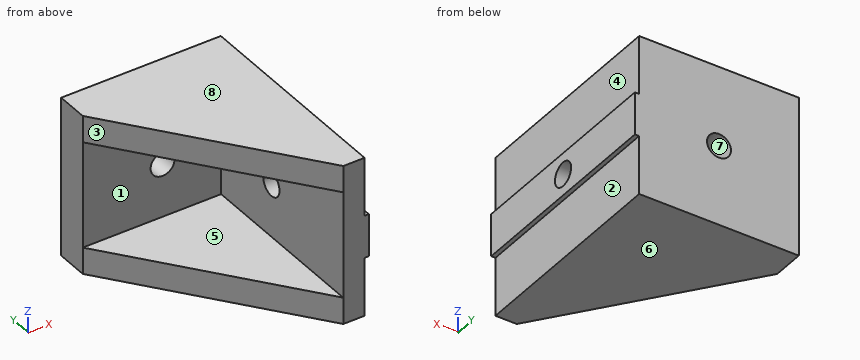
from build123d import *

# Parameters (mm, degrees)
BOSS_EXTRUDE1_DEPTH = 15
SKETCH2_W           = 8
SKETCH2_H           = 40
BOSS_EXTRUDE2_DEPTH = 0.8
SKETCH3_W           = 26
SKETCH3_H           = 34
CUT_EXTRUDE1_DEPTH  = 10
SKETCH4_R           = 2.25
CUT_EXTRUDE2_DEPTH  = 51.009999
SKETCH5_R           = 2.25
CUT_EXTRUDE3_DEPTH  = 53.201532545


with BuildPart() as part:
    # Sketch1 → Boss-Extrude1 (new, symmetric)
    with BuildSketch(Plane.XY):
        Polygon((0, 0), (-30, 0), (-30, -6), (-4, -40), (0, -40), align=None)
    extrude(amount=BOSS_EXTRUDE1_DEPTH, both=True)

    # Sketch2 → Boss-Extrude2 (add)
    with BuildSketch(Plane(origin=(0, 0, 0), x_dir=(0, 0, -1), z_dir=(1, 0, 0))):
        with Locations((0, -20)):
            Rectangle(SKETCH2_W, SKETCH2_H)
    extrude(amount=BOSS_EXTRUDE2_DEPTH)

    # Sketch3 → Cut-Extrude1 (cut, symmetric)
    with BuildSketch(Plane.XY):
        with Locations((-17, -23)):
            Rectangle(SKETCH3_W, SKETCH3_H)
    extrude(amount=CUT_EXTRUDE1_DEPTH, both=True, mode=Mode.SUBTRACT)

    # Sketch4 → Cut-Extrude2 (cut, through all)
    with BuildSketch(Plane.ZY.offset(4)):
        with Locations((0, -20)):
            Circle(SKETCH4_R)
    extrude(amount=-CUT_EXTRUDE2_DEPTH, mode=Mode.SUBTRACT)

    # Sketch5 → Cut-Extrude3 (cut, through all)
    with BuildSketch(Plane(origin=(0, 0, 0), x_dir=(1, 0, 0), z_dir=(0, 1, 0))):
        with Locations(Location((-15, 0, 0), (0, 0, 270))):
            Circle(SKETCH5_R)
    extrude(amount=-CUT_EXTRUDE3_DEPTH, mode=Mode.SUBTRACT)


solid = part.part
Input: part model. Units: mm. Frame: model coordinates. Face numbers are marked on the shaded views. A direction names the side the tool comes from. Coordinates: 2 decimals unless noted, no trailing zeros. Loops run counter-clockwise (first coordinate to the right, second up) from the corner with the lowest first, then second, coordinate; pieces in that order, holes last. Notation, with made-up numbers: (-11.75, 48) -> (31.25, 48) arc R25 ccw to (31.25, 68) -> close; hole circle Ø5 at (60.5, 38). An arc over 180 degrees is marked (long way). Write item = value, one per line. Start each with the question number.
Item 1: Cut plane D-D, the plane z = -7.25. Return loops of the section in (x, y).
Item 2: Cut plane C-C, the plane x = -15. Return loops of the section in (y, z).
Item 3: Reachability of the marked faces 1, 2, 3 and 4 from +Z, -Z, +X, -X, +Y, -Y: full face, straight path, thin tool, end or side. Return the list, or none.
Item 4: Material intervals for line 1 (X direction, y = -1.45, z = 0); line 2 (Y direction, x = -0.7, z = 0); line 3 (Z direction, x = -8, y = -31), sorted ascending.
Item 5: Mould query, pull axis Z, two halves, no side actions, for the marked faces 5, 6, 7 and 8. Classes: pulls with the +Z half, pulls with the -Z half, needs draft (parallel to the pull), parting line crosses it, or undercut.
Item 6: First-contact query: P1, Ø2.5, axis at y = -20, z = 0, coming from the -X side; P2, Ø2, axis at y = -8.5, z = -2.5, coming from the -X side; P3, Ø10, axis at x = -21, z = 2, coming from the -Y side; P4, Ø3.5, axis at y = -24.5, z = -7.5, coming from the +X side. Flat tips, straight axial feed; report the tip coordinate or a pass-through.
Item 7: Cut plane A-A, the plane z = 0. Return loops of the section in (x, y), plus the area to 3 significant figures.
Item 8: Cut plane B-B, the plane y = -21. Return loops of the section in (x, z), plus the area to 3 significant figures.
Ans:
q1.outline = (-30, -6) -> (-4, -6) -> (-4, -40) -> (0, -40) -> (0, 0) -> (-30, 0) -> close
q2.outline = (-25.62, -15) -> (0, -15) -> (0, -2.25) -> (-6, -2.25) -> (-6, -10) -> (-25.62, -10) -> close; (-25.62, 10) -> (-6, 10) -> (-6, 2.25) -> (0, 2.25) -> (0, 15) -> (-25.62, 15) -> close
q3.face_1 = -X, -Y
q3.face_2 = -Z, +X, +Y, -Y
q3.face_3 = +Z, -Z, -X, -Y
q3.face_4 = +Z, +X, +Y, -Y
q4.line_1 = -30 to -17.25, -12.75 to 0.8
q4.line_2 = -40 to -22.25, -17.75 to 0
q4.line_3 = -15 to -10, 10 to 15
q5.face_5 = undercut
q5.face_6 = pulls with the -Z half
q5.face_7 = undercut
q5.face_8 = pulls with the +Z half
q6.P1 = through
q6.P2 = -4
q6.P3 = -6
q6.P4 = 0
q7.outline = (-30, -6) -> (-17.25, -6) -> (-17.25, 0) -> (-30, 0) -> close; (-12.75, -6) -> (-4, -6) -> (-4, -17.75) -> (0.8, -17.75) -> (0.8, 0) -> (-12.75, 0) -> close; (-4, -40) -> (0.8, -40) -> (0.8, -22.25) -> (-4, -22.25) -> close
q7.area = 299 mm²
q8.outline = (-18.53, -15) -> (0, -15) -> (0, -4) -> (0.8, -4) -> (0.8, -2.02) -> (-4, -2.02) -> (-4, -10) -> (-18.53, -10) -> close; (-18.53, 10) -> (-4, 10) -> (-4, 2.02) -> (0.8, 2.02) -> (0.8, 4) -> (0, 4) -> (0, 15) -> (-18.53, 15) -> close
q8.area = 252 mm²
